```python
from build123d import *

# Parameters (mm, degrees)
SKETCH2_R          = 5
SKETCH2_R_2        = 10
CUT_EXTRUDE1_DEPTH = 26


with BuildPart() as part:
    # Sketch1 → Revolve1 (revolve)
    with BuildSketch(Plane.XY, mode=Mode.PRIVATE) as revolve1_sk:
        Polygon((-20.5, 0), (-20.5, 16), (-8.667840434, 18), (-8.667840434, 35), (-17.5, 38), (-17.5, 48), (17.5, 48), (17.5, 38), (8.667840434, 35), (8.667840434, 18), (20.5, 16), (20.5, 0), align=None)
    revolve(revolve1_sk.sketch.rotate(Axis((-20.5, 0, 0), (1, 0, 0)), 90), axis=Axis((-20.5, 0, 0), (1, 0, 0)))

    # Sketch2 → Cut-Extrude1 (cut)
    with BuildSketch(Plane.ZY.offset(8.667840434)):
        with Locations((0, 26.5)):
            Circle(SKETCH2_R)
        with Locations((26.5, 0)):
            Circle(SKETCH2_R)
        with Locations((0, -26.5)):
            Circle(SKETCH2_R)
        with Locations((-26.5, 0)):
            Circle(SKETCH2_R)
        Circle(SKETCH2_R_2)
    extrude(amount=-CUT_EXTRUDE1_DEPTH, mode=Mode.SUBTRACT)


solid = part.part
```
Check sheet for the modelled part. Datum: model origin and axes. Units: mm. A direction names the side the tool comes from. Round coordinates to 2 decimals unless told otherwise and drop trailing zeros. Loops run counter-clockwise (first coordinate to the right, second up) from the corner with the lowest first, then second, coordinate; pieces in that order, holes last. Notation, with made-up numbers: (-6.5, 47.25) - (48.5, 47.25) arc R30 ccw to (48.5, 73.25) - close; hole circle Ø9 at (83, -5). An arc over 180 degrees is marked (long way). Answer as a JSON object with one key per item and string values. Group by question number.
Q1. Set-up check for faces 1 (the face through (-8.668, 15, -15)), 2 (the face through (17.332, 0, 0)), 3 (the face through (8.668, 15, 15)), 4 (the face through (-0.12, -31.38, -1.08)): record each of +Z, -Z, +X, -X, +Y, -Y from which the full face is reachable in a straight line by a thin tool's end or side.
Q2. Gauge pin test, flat ends, axial feed: P1, Ø6, axis at x = 9.5, z = 14.5, coming from the +Y side; P2, Ø2, axis at x = -15.5, y = 7, coming from the +Z side; P3, Ø1.5, axis at x = -11.5, y = 22, coming from the -Z side. Record the tip position at first contact, or that the pin passes through.
Q3. Scan lines: line 1 along Y through (x, z) = (2.5, 0); line 2 along Z through (x, y) = (-0.5, 2); line 3 along Y through (x, z) = (10.5, 6). Record each from-to range of solid material in increasing order. Write a range as [from, to].
Q4. Mould release check, pull along Z, two halves, no side actions. Record for faces 5 (the face through (4.15, -9.76, -2.17)), 6 (the face through (-20.5, 0, 0)), 7 (the face through (0.245, -14.418, 45.783)), 8 (the face through (-0.121, 0.22, 21.505)): released by +Z, released by -Z, zero draft, split by the parting line, or undercut.
Q5. Sectioned sample at A-A, the plane z = 0. Count the separate pieces of the cut face and the enclosed holes in it, plus the area to 3 significant figures.
Q6. Sectioned sample at B-B, the plane x = 16. Enter the section's corners in (y, z), plus the area to 3 significant figures.
Solution:
{
 "1": {"face 1": "-X", "face 2": "none", "face 3": "+X", "face 4": "+X, -X"},
 "2": {"P1": "stops at y = 46.6", "P2": "stops at z = 47.62", "P3": "stops at z = -43.04"},
 "3": {"line 1": "y = [-48, -31.5], [-21.5, -10], [10, 21.5], [31.5, 48]", "line 2": "z = [-47.96, -31.08], [-21.92, -9.8], [9.8, 21.92], [31.08, 47.96]", "line 3": "y = [-47.62, -35.11], [-16.64, -8], [8, 16.64], [35.11, 47.62]"},
 "4": {"face 5": "undercut", "face 6": "zero draft", "face 7": "split by the parting line", "face 8": "undercut"},
 "5": {"separate pieces": "3", "enclosed holes": "1", "area": "2,010 mm²"},
 "6": {"outline": "circle Ø96 at (0, 0); circle Ø33.52 at (0, 0); hole circle Ø74.98 at (0, 0); hole circle Ø20 at (0, 0)", "area": "3,390 mm²"}
}
